Here's how the part is built. I have some questions about the finished solid (model axes, mm). Give positions to 0.01 mm unless a question says otherwise; leave off trailing zeros. Write each loop counter-clockwise with the first axis right and the second up, starting at its lowest first coordinate (ties: lowest second). Pieces come first, ordered by that corner, then holes. Notation, with made-up numbers: (-9.5, 48.5) - (17.5, 48.5) arc R21 ccw to (17.5, 66.5) - close; hole circle Ø11 at (48, -22). An arc over 180 degrees is marked (long way). One line per item, written item: value. Start each with the question number.
1) Imagine slicing it at C-C on y = 317. Write out the boundary of the cut face in (x, z).
2) Please list where these lines run through material, in increasing order: L1, parallel to Y at x = 640, z = 20; L2, parallel to Z at x = 637, y = 166.5; L3, parallel to Z at x = 639, y = 166. Write a range as [from, to].
3) Imagine slicing it at A-A on z = -13. Count the separate pieces of the cut face and the enclosed holes in it, plus the area to 3 significant figures.
4) I'm going to push flat-ended pins straight in: P1, Ø3, axis at x = 649.5, y = 143, coming from the +Z side; P2, Ø6, axis at x = 640, z = -19.5, coming from the +Y side; P3, Ø4, axis at y = 150, z = 23.5, coming from the +X side. Where does each tip first touch, or does it pass through?
5) Imagine slicing it at B-B on y = 187. Write out the boundary of the cut face in (x, z).
from build123d import *

# Parameters (mm, degrees)
SKETCH1_R                = 34.544
BOSS_EXTRUDE1_DEPTH      = 6.35
BOSS_EXTRUDE1_DEPTH_BACK = 12.7
CUT_EXTRUDE1_START       = -12.7
SKETCH2_W                = 38.1
SKETCH2_H                = 25.4
CUT_EXTRUDE1_DEPTH       = 12.7
SKETCH3_R                = 39.3065
SKETCH3_R_2              = 34.544
BOSS_EXTRUDE2_DEPTH      = 17.526
SKETCH4_R                = 34.544
SKETCH4_R_2              = 28.194
BOSS_EXTRUDE3_DEPTH      = 1.5875


with BuildPart() as part:
    # Sketch1 → Boss-Extrude1 (new body, two sides)
    with BuildSketch(Plane(origin=(648.29757997, 2.828749778, 0), x_dir=(0, 0, -1), z_dir=(0.999990481, 0.004363309, 0))) as boss_extrude1_sk:
        with BuildLine():
            Line((10.162421384, 149.738796817), (10.162421384, 124.338796817))
            Line((10.162421384, 124.338796817), (-27.937578616, 124.338796817))
            Line((-27.937578616, 124.338796817), (-27.937578616, 149.738796817))
            Line((-27.937578616, 149.738796817), (-38.969975232, 233.506353672))
            ThreePointArc((-38.969975232, 233.506353672), (-38.774533686, 245.083676928), (-35.214302621, 256.101724211))
            Line((-35.214302621, 256.101724211), (-12.384316038, 302.138796817))
            Line((-12.384316038, 302.138796817), (-12.384316038, 327.538796817))
            Line((-12.384316038, 327.538796817), (25.715683962, 327.538796817))
            Line((25.715683962, 327.538796817), (25.715683962, 302.138796817))
            Line((25.715683962, 302.138796817), (38.304504923, 247.457291294))
            ThreePointArc((38.304504923, 247.457291294), (39.241875136, 236.385759301), (37.043517063, 225.49426237))
            Line((37.043517063, 225.49426237), (10.162421384, 149.738796817))
        make_face()
        with Locations((0, 238.638796817)):
            Circle(SKETCH1_R, mode=Mode.SUBTRACT)
        with BuildLine():
            Line((22.400354986, 295.311648337), (29.455908243, 264.664753318))
            ThreePointArc((29.455908243, 264.664753318), (19.813317438, 272.586306215), (8.173615245, 277.086071832))
            Line((8.173615245, 277.086071832), (22.400354986, 295.311648337))
        make_face(mode=Mode.SUBTRACT)
        with BuildLine():
            Line((-1.363444644, 277.921642449), (-10.508730274, 295.201256573))
            Line((-10.508730274, 295.201256573), (-22.615671737, 270.787394518))
            ThreePointArc((-22.615671737, 270.787394518), (-12.508951954, 275.901741725), (-1.363444644, 277.921642449))
        make_face(mode=Mode.SUBTRACT)
        Polygon((19.984225718, 297.376296817), (3.266942404, 275.960137419), (-8.067621746, 297.376296817), align=None, mode=Mode.SUBTRACT)
        with BuildLine():
            Line((26.283654933, 209.412602647), (8.894198101, 160.406177697))
            Line((8.894198101, 160.406177697), (-1.749435192, 199.371247635))
            ThreePointArc((-1.749435192, 199.371247635), (13.254779787, 201.63458415), (26.283654933, 209.412602647))
        make_face(mode=Mode.SUBTRACT)
        with BuildLine():
            Line((-5.104730105, 199.665181732), (-24.520278978, 160.264997004))
            Line((-24.520278978, 160.264997004), (-31.799445858, 215.534767182))
            ThreePointArc((-31.799445858, 215.534767182), (-20.085828001, 204.851810331), (-5.104730105, 199.665181732))
        make_face(mode=Mode.SUBTRACT)
        Polygon((-3.852902363, 195.022655751), (7.215844228, 154.501296817), (-23.820941352, 154.501296817), align=None, mode=Mode.SUBTRACT)
    extrude(amount=BOSS_EXTRUDE1_DEPTH)
    extrude(boss_extrude1_sk.sketch, amount=-BOSS_EXTRUDE1_DEPTH_BACK)

    # Sketch2 → Cut-Extrude1 (cut)
    with BuildSketch(Plane(origin=(635.597700865, 2.77333575, 0), x_dir=(0, 0, 1), z_dir=(-0.999990481, -0.004363309, 0)).offset(CUT_EXTRUDE1_START)):
        with Locations((-6.665683962, 314.838796817)):
            Rectangle(SKETCH2_W, SKETCH2_H)
        with Locations((8.887578616, 137.038796817)):
            Rectangle(SKETCH2_W, SKETCH2_H)
    extrude(amount=CUT_EXTRUDE1_DEPTH, mode=Mode.SUBTRACT)

    # Sketch3 → Boss-Extrude2 (add)
    with BuildSketch(Plane(origin=(635.597700865, 2.77333575, 0), x_dir=(0, 0, 1), z_dir=(-0.999990481, -0.004363309, 0))):
        with Locations((0, 238.638796817)):
            Circle(SKETCH3_R)
        with Locations((0, 238.638796817)):
            Circle(SKETCH3_R_2, mode=Mode.SUBTRACT)
    extrude(amount=BOSS_EXTRUDE2_DEPTH)

    # Sketch4 → Boss-Extrude3 (add, symmetric)
    with BuildSketch(Plane(origin=(636.359693611, 2.776660591, 0), x_dir=(0, 0, 1), z_dir=(-0.999990481, -0.004363309, 0))):
        with Locations((0, 238.638796817)):
            Circle(SKETCH4_R)
        with Locations((0, 238.638796817)):
            Circle(SKETCH4_R_2, mode=Mode.SUBTRACT)
    extrude(amount=BOSS_EXTRUDE3_DEPTH, both=True)


solid = part.part
Numbers:
1. outline: (646.93, -25.72) - (653.28, -25.72) - (653.28, 12.38) - (646.93, 12.38) - close
2. L1: [152.53, 157.3], [165.05, 172.23], [207.6, 213.27], [269.6, 275.27], [278.86, 289.58]
2. L2: [-15.12, -10.07], [-7.99, -4.7], [19.28, 22.82], [24.98, 29.78]
2. L3: [-14.94, -9.89], [-8.13, -4.84], [19.53, 23.07], [24.91, 29.71]
3. separate pieces: 5
3. enclosed holes: 0
3. area: 1,040 mm^2
4. P1: z = 27.94
4. P2: y = 304.95
4. P3: x = 654.01
5. outline: (634.79, -22.4) - (653.84, -22.37) - (653.84, -17.32) - (634.79, -17.35) - close; (634.79, -2.39) - (653.84, -2.41) - (653.84, 0.88) - (634.79, 0.9) - close; (634.79, 9.17) - (653.84, 9.21) - (653.84, 12.75) - (634.79, 12.71) - close; (634.79, 27.68) - (653.84, 27.67) - (653.84, 32.47) - (634.79, 32.48) - close
